Can you work these out from the model? Positions are in its coordinate system, mm. A direction names the side the tool comes from. Coordinates: 2 decimals unless noted, no trailing zeros. Write each loop counter-clockwise with the first axis right and the second up, starting at its lowest first coordinate (ties: lowest second). Pieces come first, ordered by that corner, then holes. Notation, with made-up numbers: M -10,-35.5 L 38,-35.5 A15 cw 38,-19.5 Z; hole C -4.75,69.5 d9. An arc over 180 degrees is marked long. Use one line per item in the form item = value. Start each with the question number.
```python
from build123d import *

# Parameters (mm, degrees)
F1_DEPTH = 9.5
F0_R     = 2.7
F2_DEPTH = 12.75
F3_DEPTH = 0.5


with BuildPart() as f1:
    # F0 (on Top) → F1 (new body, symmetric)
    with BuildSketch(Plane.XY):
        with BuildLine():
            Line((10.9217294241, 6.0799529679), (10.9217294241, 7.9351009059))
            Line((10.9217294241, 7.9351009059), (9.1573788889, 8.5083731459))
            ThreePointArc((9.1573788889, 8.5083731459), (10.1127124848, 7.3473156937), (10.9217294241, 6.0799529679))
        make_face()
        with BuildLine():
            ThreePointArc((12.5000000682, 0), (12.0990003771, 3.1407310581), (10.9217294241, 6.0799529679))
            Line((10.9217294241, 6.0799529679), (10.9217294241, 0))
            Line((10.9217294241, 0), (10.9217294241, -6.0799529679))
            ThreePointArc((10.9217294241, -6.0799529679), (12.0990003771, -3.1407310581), (12.5000000682, 0))
        make_face()
        with BuildLine():
            Line((10.9217294241, 0), (10.9217294241, 6.0799529679))
            ThreePointArc((10.9217294241, 6.0799529679), (10.1127124848, 7.3473156937), (9.1573788889, 8.5083731459))
            Line((9.1573788889, 8.5083731459), (3.3749999593, 10.3871819512))
            ThreePointArc((3.3749999593, 10.3871819512), (8.8358646995, 6.4196315023), (10.9217294241, 0))
        make_face()
        with BuildLine():
            Line((3.3749999593, 10.3871819512), (9.1573788889, 8.5083731459))
            ThreePointArc((9.1573788889, 8.5083731459), (3.8627124507, 11.8882065185), (-2.4073788889, 12.26599073))
            Line((-2.4073788889, 12.26599073), (3.3749999593, 10.3871819512))
        make_face()
        with BuildLine():
            Line((10.9217294241, -6.0799529679), (10.9217294241, 0))
            ThreePointArc((10.9217294241, 0), (8.8358646995, -6.4196315023), (3.3749999593, -10.3871819512))
            Line((3.3749999593, -10.3871819512), (9.1573788889, -8.5083731459))
            ThreePointArc((9.1573788889, -8.5083731459), (10.1127124848, -7.3473156937), (10.9217294241, -6.0799529679))
        make_face()
        with BuildLine():
            ThreePointArc((-8.8358646984, 6.4196315037), (-3.3750000093, 10.3871819349), (3.3749999593, 10.3871819512))
            Line((3.3749999593, 10.3871819512), (-2.4073788889, 12.26599073))
            ThreePointArc((-2.4073788889, 12.26599073), (-3.8627124507, 11.8882065185), (-5.2621580229, 11.338416761))
            Line((-5.2621580229, 11.338416761), (-8.8358646984, 6.4196315037))
        make_face()
        with BuildLine():
            ThreePointArc((-5.2621580229, 11.338416761), (-3.8627124507, 11.8882065185), (-2.4073788889, 12.26599073))
            Line((-2.4073788889, 12.26599073), (-4.1717294241, 12.83926297))
            Line((-4.1717294241, 12.83926297), (-5.2621580229, 11.338416761))
        make_face()
        with BuildLine():
            Line((10.9217294241, -7.9351009059), (10.9217294241, -6.0799529679))
            ThreePointArc((10.9217294241, -6.0799529679), (10.1127124848, -7.3473156937), (9.1573788889, -8.5083731459))
            Line((9.1573788889, -8.5083731459), (10.9217294241, -7.9351009059))
        make_face()
        with BuildLine():
            Line((9.1573788889, -8.5083731459), (3.3749999593, -10.3871819512))
            Line((3.3749999593, -10.3871819512), (-2.4073788889, -12.26599073))
            ThreePointArc((-2.4073788889, -12.26599073), (3.8627124507, -11.8882065185), (9.1573788889, -8.5083731459))
        make_face()
        with BuildLine():
            Line((-2.4073788889, -12.26599073), (3.3749999593, -10.3871819512))
            ThreePointArc((3.3749999593, -10.3871819512), (-3.3749999125, -10.3871819664), (-8.8358645787, -6.4196316685))
            Line((-8.8358645787, -6.4196316685), (-5.2621580229, -11.338416761))
            ThreePointArc((-5.2621580229, -11.338416761), (-3.8627124507, -11.8882065185), (-2.4073788889, -12.26599073))
        make_face()
        with BuildLine():
            ThreePointArc((-8.8358645787, -6.4196316685), (-10.9217294241, -1.018e-07), (-8.8358646984, 6.4196315037))
            Line((-8.8358646984, 6.4196315037), (-12.4095714012, 1.500846209))
            ThreePointArc((-12.4095714012, 1.500846209), (-12.5000000682, 0), (-12.4095714012, -1.500846209))
            Line((-12.4095714012, -1.500846209), (-8.8358645787, -6.4196316685))
        make_face()
        with BuildLine():
            Line((-12.4095714012, 1.500846209), (-8.8358646984, 6.4196315037))
            Line((-8.8358646984, 6.4196315037), (-5.2621580229, 11.338416761))
            ThreePointArc((-5.2621580229, 11.338416761), (-10.1127124848, 7.3473156937), (-12.4095714012, 1.500846209))
        make_face()
        with BuildLine():
            Line((-4.1717294241, -12.83926297), (-2.4073788889, -12.26599073))
            ThreePointArc((-2.4073788889, -12.26599073), (-3.8627124507, -11.8882065185), (-5.2621580229, -11.338416761))
            Line((-5.2621580229, -11.338416761), (-4.1717294241, -12.83926297))
        make_face()
        with BuildLine():
            Line((-5.2621580229, -11.338416761), (-8.8358645787, -6.4196316685))
            Line((-8.8358645787, -6.4196316685), (-12.4095714012, -1.500846209))
            ThreePointArc((-12.4095714012, -1.500846209), (-10.1127124848, -7.3473156937), (-5.2621580229, -11.338416761))
        make_face()
        with BuildLine():
            ThreePointArc((-12.4095714012, -1.500846209), (-12.5000000682, 0), (-12.4095714012, 1.500846209))
            Line((-12.4095714012, 1.500846209), (-13.5, 0))
            Line((-13.5, 0), (-12.4095714012, -1.500846209))
        make_face()
    extrude(amount=F1_DEPTH, both=True)



with BuildPart() as f1b:
    # F0 (on Top) → F1, piece 2 (new body, symmetric)
    with BuildSketch(Plane.XY):
        Circle(F0_R)
    extrude(amount=F1_DEPTH, both=True)

    # F0 (on Top) → F2 (join, symmetric)
    with BuildSketch(Plane.XY):
        Circle(F0_R)
    extrude(amount=F2_DEPTH, both=True)


with BuildPart() as f1_1:
    add(f1.part)

    add(f1b.part)  # F3 merges F1b
    # F0 (on Top) → F3 (join, symmetric)
    with BuildSketch(Plane.XY):
        with BuildLine():
            ThreePointArc((3.3749999593, -10.3871819512), (8.8358646995, -6.4196315023), (10.9217294241, 0))
            ThreePointArc((10.9217294241, 0), (8.8358646995, 6.4196315023), (3.3749999593, 10.3871819512))
            ThreePointArc((3.3749999593, 10.3871819512), (-3.3750000093, 10.3871819349), (-8.8358646984, 6.4196315037))
            ThreePointArc((-8.8358646984, 6.4196315037), (-10.9217294241, -1.018e-07), (-8.8358645787, -6.4196316685))
            ThreePointArc((-8.8358645787, -6.4196316685), (-3.3749999125, -10.3871819664), (3.3749999593, -10.3871819512))
        make_face()
        Circle(F0_R, mode=Mode.SUBTRACT)
    extrude(amount=F3_DEPTH, both=True)


solid = f1_1.part
```
1) Suppose I cut it at A-A on z = -8. Please give me the cut outline in (x, y) (3 decimals), and give its area (3 significant figures).
2) If we mould it in two halves opening along Y, with no side actions, what happens to faces 1 (the face through (-0.585, -2.636, -6.539)), 2 (the face through (-3.302, -12.557, 0.133)), 3 (the face through (2.3, -2.3, 0.5)), 4 (the face through (0, 0, -12.75))? For each: +Y half, -Y half, draft (parallel to the pull), parting line (faces both ways), or undercut.
3) Will these pins go through, and if not, where does the flat tip stop? pin 1 Ø3 at (y, z) = (-2.5, -4.5) entering from +X; pin 2 Ø12 at (x, y) = (-1, -9) entering from -Z; pin 3 Ø1.5 at (y, z) = (-7, 1.5) entering from +X.
4) Please list where these lines run through material, in increasing order: line 1 (Y direction, x = 0.5, z = -1); line 2 (Y direction, x = 2, z = -7.5); line 3 (Z direction, x = -8.5, y = -8.75).
5) Suppose I cut it at C-C on y = 4. Please give me the cut outline in (x, z).
6) Which directions (+Z, -Z, +X, -X, +Y, -Y) give clear straight access to the entire face, cutting with the end or side of a thin tool? Please do faces 5 (the face through (-3.28, 12.55, 0.13)), 6 (the face through (10.922, -7, 0)), 7 (the face through (10.922, 7, 0)).
7) Suppose I cut it at D-D on x = -6.5. Please give me the cut outline in (y, z).
8) Suppose I cut it at B-B on x = 0. Please give me the cut outline in (y, z).
Computed values:
q1.outline = M -13.5,0 L -12.41,-1.501 A12.5 ccw -5.262,-11.338 L -4.172,-12.839 L -2.407,-12.266 A12.5 ccw 9.157,-8.508 L 10.922,-7.935 L 10.922,-6.08 A12.5 ccw 10.922,6.08 L 10.922,7.935 L 9.157,8.508 A12.5 ccw -2.407,12.266 L -4.172,12.839 L -5.262,11.338 A12.5 ccw -12.41,1.501 Z; C 0,0 d5.4; hole C 0,0 d21.843
q1.area = 146 mm²
q2.face_1 = undercut
q2.face_2 = -Y half
q2.face_3 = undercut
q2.face_4 = draft
q3.pin_1 = 12.46
q3.pin_2 = -9.5
q3.pin_3 = 10.92
q4.line_1 = -12.49 to -10.91, -2.65 to 2.65, 10.91 to 12.49
q4.line_2 = -12.34 to -10.74, -1.81 to 1.81, 10.74 to 12.34
q4.line_3 = -9.5 to 9.5
q5.outline = M -11.84,-9.5 L -10.16,-9.5 L -10.16,-0.5 L 10.16,-0.5 L 10.16,-9.5 L 11.84,-9.5 L 11.84,9.5 L 10.16,9.5 L 10.16,0.5 L -10.16,0.5 L -10.16,9.5 L -11.84,9.5 Z
q6.face_5 = +Z, -Z, +Y
q6.face_6 = +Z, -Z, +X, -Y
q6.face_7 = +Z, -Z, +X, +Y
q7.outline = M -10.68,-9.5 L -8.78,-9.5 L -8.78,-0.5 L 8.78,-0.5 L 8.78,-9.5 L 10.68,-9.5 L 10.68,9.5 L 8.78,9.5 L 8.78,0.5 L -8.78,0.5 L -8.78,9.5 L -10.68,9.5 Z
q8.outline = M -12.5,-9.5 L -10.92,-9.5 L -10.92,-0.5 L -2.7,-0.5 L -2.7,-12.75 L 2.7,-12.75 L 2.7,-0.5 L 10.92,-0.5 L 10.92,-9.5 L 12.5,-9.5 L 12.5,9.5 L 10.92,9.5 L 10.92,0.5 L 2.7,0.5 L 2.7,12.75 L -2.7,12.75 L -2.7,0.5 L -10.92,0.5 L -10.92,9.5 L -12.5,9.5 Z
